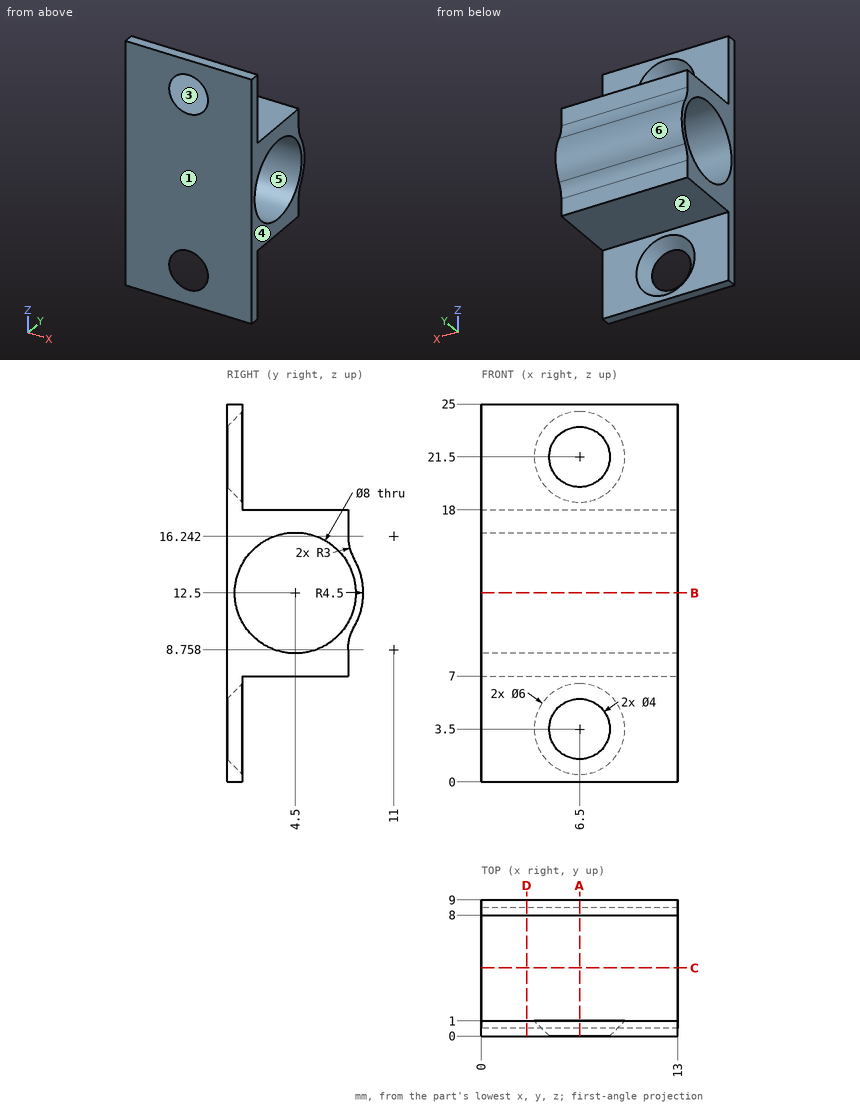
Source: three-view drawing plus pictorial views. Frame: mm from the lowest corner of the part. A direction names the side the tool comes from. Coordinates: 2 decimals unless noted, no trailing zeros. Write each loop counter-clockwise with the first axis right and the second up, starting at its lowest first coordinate (ties: lowest second). Pieces come first, ordered by that corner, then holes. Notation, with made-up numbers: (-30.5, 69) -> (-6.5, 69) arc R15 ccw to (-6.5, 94) -> close; hole circle Ø1 at (32.25, 35). An arc over 180 degrees is marked (long way). Answer as a JSON object with one key per item and string values.
1. Access query for the marked faces 1, 2 and 3. Directions: +Z, -Z, +X, -X, +Y, -Y. A direction counts if a zero-diameter tool reaches every point of the face in a straight line with its end or side. Return the directions, or none.
Result set:
{"face 1": "+Z, -Z, +X, -X, -Y", "face 2": "-Z, +X, -X, +Y", "face 3": "+Z, +X, -X, +Y"}
2. Section A-A on x = 6.5. Return the cut outline in (y, z) (1 decimal).
Result set:
{"outline": "(0, 0) -> (1, 0) -> (1, 0.5) -> (0, 1.5) -> close; (0, 5.5) -> (1, 6.5) -> (1, 7) -> (8, 7) -> (8, 8.8) arc R3 cw to (8.4, 10.3) arc R4.5 ccw to (8.4, 14.7) arc R3 cw to (8, 16.2) -> (8, 18) -> (1, 18) -> (1, 18.5) -> (0, 19.5) -> close; (0, 23.5) -> (1, 24.5) -> (1, 25) -> (0, 25) -> close; hole circle Ø8 at (4.5, 12.5)"}
3. Section D-D on x = 3. Return the cut outline in (y, z) (1 decimal).
Result set:
{"outline": "(0, 0) -> (1, 0) -> (1, 7) -> (8, 7) -> (8, 8.8) arc R3 cw to (8.4, 10.3) arc R4.5 ccw to (8.4, 14.7) arc R3 cw to (8, 16.2) -> (8, 18) -> (1, 18) -> (1, 25) -> (0, 25) -> close; hole circle Ø8 at (4.5, 12.5)"}
4. First-contact query: P1, Ø0.5, axis at x = 6.5, z = 17, coming from the +Y side; P2, Ø5.5, axis at x = 5, z = 21, coming from the +Y side; P3, Ø2, axis at x = 7.5, z = 8.5, coming from the -Y side; P4, Ø3.5, axis at x = 5, y = 5.5, coming from the -Z side. Flat tips, straight axial feed; report the tip coordinate or a pass-through.
Result set:
{"P1": "stops at y = 8", "P2": "stops at y = 1", "P3": "stops at y = 0", "P4": "stops at z = 7"}
5. Section B-B on z = 12.5. Return the cut outline in (x, y), then the cut area to 3 significant figures.
Result set:
{"outline": "(0, 0) -> (13, 0) -> (13, 0.5) -> (0, 0.5) -> close; (0, 8.5) -> (13, 8.5) -> (13, 9) -> (0, 9) -> close", "area": "13.0 mm2"}
6. Section C-C on y = 4.5. Return the cut outline in (x, z).
Result set:
{"outline": "(0, 7) -> (13, 7) -> (13, 8.5) -> (0, 8.5) -> close; (0, 16.5) -> (13, 16.5) -> (13, 18) -> (0, 18) -> close"}
7. Material intervals for line 1 (Y direction, x = 10.5, z = 12.5); line 2 (Y direction, x = 4.5, z = 5); line 3 (Z direction, x = 7.5, y = 7), sorted ascending. Write a range as from..to.
Result set:
{"line 1": "y = 0..0.5, 8.5..9", "line 2": "y = 0..0.5", "line 3": "z = 7..9.38, 15.62..18"}
8. Mould query, pull axis Z, two halves, no side actions, for the marked faces 4, 5 and 6. Classes: released by +Z, released by -Z, zero draft, split by the parting line, or undercut.
Result set:
{"face 4": "zero draft", "face 5": "undercut", "face 6": "split by the parting line"}
